from build123d import *

# Parameters (mm, degrees)
SKETCH1_W           = 12.7
SKETCH1_H           = 12.7
BOSS_EXTRUDE1_DEPTH = 15.24
SKETCH2_W           = 6.35
SKETCH2_H           = 7.62
CUT_EXTRUDE1_DEPTH  = 6.35
SKETCH3_W           = 3.302040176
SKETCH3_H           = 3.302040176
CUT_EXTRUDE2_DEPTH  = 5.08


with BuildPart() as part:
    # Sketch1 → Boss-Extrude1 (new body)
    with BuildSketch(Plane.XY):
        Rectangle(SKETCH1_W, SKETCH1_H)
    extrude(amount=BOSS_EXTRUDE1_DEPTH)

    # Sketch2 → Cut-Extrude1 (cut)
    with BuildSketch(Plane.XY.offset(15.24)):
        with Locations((0, 2.54)):
            Rectangle(SKETCH2_W, SKETCH2_H)
    extrude(amount=-CUT_EXTRUDE1_DEPTH, mode=Mode.SUBTRACT)

    # Sketch3 → Cut-Extrude2 (cut)
    with BuildSketch(Plane(origin=(0, 0, 0), x_dir=(-1, 0, 0), z_dir=(0, 0, -1))):
        Rectangle(SKETCH3_W, SKETCH3_H)
    extrude(amount=-CUT_EXTRUDE2_DEPTH, mode=Mode.SUBTRACT)


solid = part.part
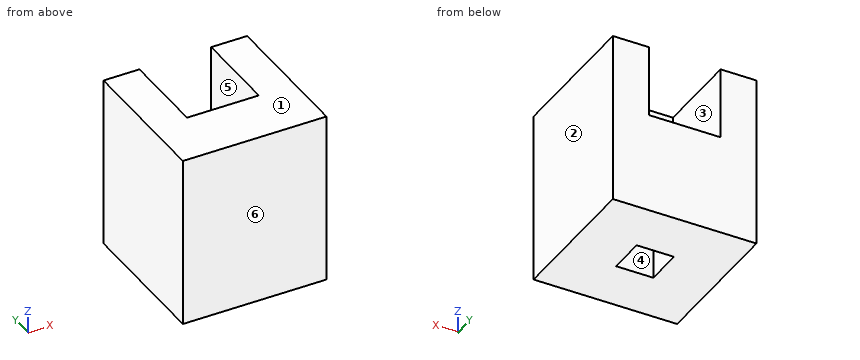
Can you work these out from the model? Positions are in its coordinate system, mm. Face numbers are marked on the shaded views. A direction names the side the tool comes from. Coordinates: 2 decimals unless noted, no trailing zeros. Write each loop counter-clockwise with the first axis right and the second up, starting at its lowest first coordinate (ties: lowest second). Pieces come first, ordered by that corner, then holes. Notation, with made-up numbers: (72.5, 63.5) -> (89.5, 63.5) arc R9 ccw to (89.5, 70.5) -> close; hole circle Ø2 at (-39.5, 36.25). An arc over 180 degrees is marked (long way). Write each question's results on one line, items separated by ' | '. Start each with the question number.
Item 1: If we section it at A-A, the plane y = 2.5: Write out the boundary of the cut face in (x, z) (3 decimals).
Item 2: If we section it at D-D, the plane y = 1: Write out the boundary of the cut face in (x, z) (3 decimals), and give its area (3 significant figures).
Item 3: If we section it at B-B, the plane z = 3.75: Write out the boundary of the cut face in (x, y).
Item 4: Thinking about a two-plate mould opening in X: for the marked faces 1, 2 and 3, which applies, released by +X, released by -X, zero draft, split by the parting line, or undercut?
Item 5: Please list where these lines run through material, in increasing order: probe 1 along X at (y, z) = (3.5, 9) (3 decimals); probe 2 along Y at (x, z) = (1.75, 14); probe 3 along Z at (x, y) = (1, 0.5).
Item 6: I'm going to push flat-ended pins straight in: P1, Ø1.5, axis at x = -4.5, y = 2, coming from the -Z side; P2, Ø3, axis at x = -0.5, y = 1.5, coming from the +Z side. Where does each tip first touch, or does it pass through?
Item 7: On a 3-axis mill with a long thin cutter (end or side, diameter ignored), from which of +Z, -Z, +X, -X, +Y, -Y can I reach the whole of each face in a straight line? I mean the marked faces 4, 5 and 6. Say none if no direction works.
Item 8: If we section it at C-C, the plane z = 11.5: Write out the boundary of the cut face in (x, y) (3 decimals).
Answer block:
1) outline: (-6.35, 0) -> (6.35, 0) -> (6.35, 15.24) -> (3.175, 15.24) -> (3.175, 8.89) -> (-3.175, 8.89) -> (-3.175, 15.24) -> (-6.35, 15.24) -> close
2) outline: (-6.35, 0) -> (-1.651, 0) -> (-1.651, 5.08) -> (1.651, 5.08) -> (1.651, 0) -> (6.35, 0) -> (6.35, 15.24) -> (3.175, 15.24) -> (3.175, 8.89) -> (-3.175, 8.89) -> (-3.175, 15.24) -> (-6.35, 15.24) -> close | area: 136 mm²
3) outline: (-6.35, -6.35) -> (6.35, -6.35) -> (6.35, 6.35) -> (-6.35, 6.35) -> close; hole (-1.65, -1.65) -> (1.65, -1.65) -> (1.65, 1.65) -> (-1.65, 1.65) -> close
4) face 1: zero draft | face 2: released by +X | face 3: undercut
5) probe 1: -6.35 to -3.175, 3.175 to 6.35 | probe 2: -6.35 to -1.27 | probe 3: 5.08 to 8.89
6) P1: z = 0 | P2: z = 8.89
7) face 4: -Z | face 5: +Z, +Y | face 6: +Z, -Z, +X, -X, -Y
8) outline: (-6.35, -6.35) -> (6.35, -6.35) -> (6.35, 6.35) -> (3.175, 6.35) -> (3.175, -1.27) -> (-3.175, -1.27) -> (-3.175, 6.35) -> (-6.35, 6.35) -> close
